```python
from build123d import *

# Parameters (mm, degrees)
BOSS_EXTRUDE1_DEPTH                             = 6.35
SKETCH2_R                                       = 9.525
MOTOR_SHAFT_HOLES_DEPTH                         = 135.10382172
SKETCH3_R                                       = 14.2875
FIRST_BEARING_HOLE_DEPTH                        = 135.10382172
SKETCH4_R                                       = 12.7
PINION_CLEARANCE_DEPTH                          = 3.175
SKETCH5_R                                       = 14.2875
CUT_EXTRUDE1_DEPTH                              = 135.10382172
CBORE_FOR_10_SOCKET_HEAD_CAP_SCREW1_D           = 5.1054
CBORE_FOR_10_SOCKET_HEAD_CAP_SCREW1_CBORE_D     = 9.525
CBORE_FOR_10_SOCKET_HEAD_CAP_SCREW1_CBORE_DEPTH = 4.826
F_10_CLEARANCE_HOLE1_D                          = 5.1054
FILLET1_R                                       = 6.35
SKETCH11_R                                      = 4.7625
CUT_EXTRUDE2_DEPTH                              = 50.8


with BuildPart() as part:
    # Sketch1 → Boss-Extrude1 (new body)
    with BuildSketch(Plane(origin=(0, 0, 0), x_dir=(1, 0, 0), z_dir=(0, 1, 0))):
        Polygon((69.85, -19.05), (69.85, 57.15), (6.35, 114.3), (-6.35, 114.3), (-69.85, 57.15), (-69.85, -19.05), align=None)
    extrude(amount=BOSS_EXTRUDE1_DEPTH)

    # Sketch2 → Motor Shaft Holes (cut, through all)
    with BuildSketch(Plane(origin=(0, 6.35, 0), x_dir=(1, 0, 0), z_dir=(0, 1, 0))):
        with Locations(Location((-34.29, 25.4, 0), (0, 0, 270))):
            Circle(SKETCH2_R)
        with Locations(Location((34.29, 25.4, 0), (0, 0, 270))):
            Circle(SKETCH2_R)
    extrude(amount=-MOTOR_SHAFT_HOLES_DEPTH, mode=Mode.SUBTRACT)

    # Sketch3 → First Bearing Hole (cut, through all)
    with BuildSketch(Plane(origin=(0, 6.35, 0), x_dir=(1, 0, 0), z_dir=(0, 1, 0))):
        with Locations(Location((0, 25.4, 0), (0, 0, 270))):
            Circle(SKETCH3_R)
    extrude(amount=-FIRST_BEARING_HOLE_DEPTH, mode=Mode.SUBTRACT)

    # Sketch4 → Pinion Clearance (cut)
    with BuildSketch(Plane(origin=(0, 6.35, 0), x_dir=(1, 0, 0), z_dir=(0, 1, 0))):
        with Locations(Location((-34.29, 25.4, 0), (0, 0, 270))):
            Circle(SKETCH4_R)
        with Locations(Location((34.29, 25.4, 0), (0, 0, 270))):
            Circle(SKETCH4_R)
    extrude(amount=-PINION_CLEARANCE_DEPTH, mode=Mode.SUBTRACT)

    # Sketch5 → Cut-Extrude1 (cut, through all)
    with BuildSketch(Plane(origin=(0, 6.35, 0), x_dir=(1, 0, 0), z_dir=(0, 1, 0))):
        with Locations(Location((0, 63.5, 0), (0, 0, 270))):
            Circle(SKETCH5_R)
    extrude(amount=-CUT_EXTRUDE1_DEPTH, mode=Mode.SUBTRACT)

    # CBORE for #10 Socket Head Cap Screw1 (through all)
    with Locations(Plane(origin=(0, 6.35, 0), x_dir=(1, 0, 0), z_dir=(0, 1, 0))):
        with Locations((-42.97731164, 49.268192568), (-25.60268836, 1.531807432)):
            cbore_for_10_socket_head_cap_screw1 = CounterBoreHole(CBORE_FOR_10_SOCKET_HEAD_CAP_SCREW1_D / 2, CBORE_FOR_10_SOCKET_HEAD_CAP_SCREW1_CBORE_D / 2, CBORE_FOR_10_SOCKET_HEAD_CAP_SCREW1_CBORE_DEPTH)

    # Mirror1: CBORE for #10 Socket Head Cap Screw1 across plane
    add(cbore_for_10_socket_head_cap_screw1.mirror(Plane(origin=(0, 0, 0), x_dir=(0, 0, 1), z_dir=(1, 0, 0))), mode=Mode.SUBTRACT)

    # #10 Clearance Hole1 (through all)
    with Locations(Plane(origin=(0, 34.925, 19.05), x_dir=(1, 0, 0), z_dir=(0, 1, 0))):
        with Locations((-63.5, 6.35), (63.5, 6.35), (0, 107.95)):
            Hole(F_10_CLEARANCE_HOLE1_D / 2)

    # Fillet1
    fillet1_edges = [part.edges().sort_by_distance(p)[0] for p in [
        (69.85, 3.175, -57.15),
        (69.85, 3.175, 19.05),
        (-69.85, 3.175, 19.05),
        (-69.85, 3.175, -57.15),
        (-6.35, 3.175, -114.3),
        (6.35, 3.175, -114.3),
    ]]
    fillet(fillet1_edges, radius=FILLET1_R)

    # Sketch11 → Cut-Extrude2 (cut)
    with BuildSketch(Plane(origin=(0, 0, 19.05), x_dir=(-1, 0, 0), z_dir=(0, -1, 0))):
        with Locations(Location((-44.45, 85.725, 0), (0, 0, 90))):
            Circle(SKETCH11_R)
        with Locations(Location((44.45, 85.725, 0), (0, 0, 90))):
            Circle(SKETCH11_R)
        with Locations(Location((0, 6.35, 0), (0, 0, 90))):
            Circle(SKETCH11_R)
    extrude(amount=-CUT_EXTRUDE2_DEPTH, mode=Mode.SUBTRACT)


solid = part.part
```
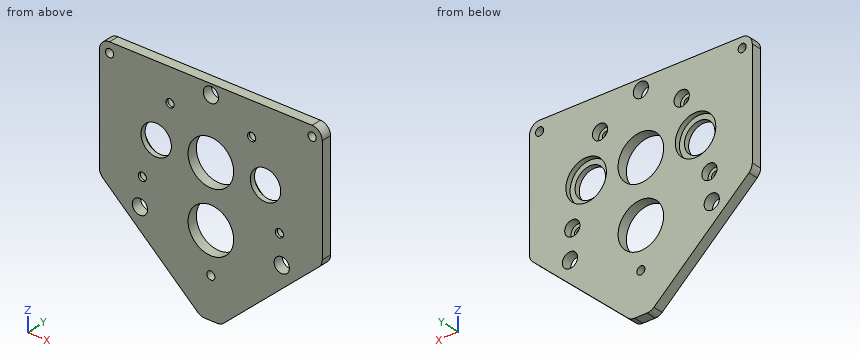
Geometry check sheet. Reference: the model listing, model coordinates, mm. Round coordinates to 2 decimals unless told otherwise and drop trailing zeros. Loops run counter-clockwise (first coordinate to the right, second up) from the corner with the lowest first, then second, coordinate; pieces in that order, holes last. Notation, with made-up numbers: M 62,60.5 L 103,60.5 A28 ccw 103,97.5 Z; hole C -18.75,46 d6. An arc over 180 degrees is marked long. Return JSON: item names as keys, results as strings. Group by question number.
(1) Go/stop test with flat-tipped pins: pin 1 (1 mm diameter, centred on x = 35, y = 1, fed in from -Z) (3 decimals); pin 2 (4.5 mm diameter, centred on x = -25.6, z = -1.53, fed in from -Y); pin 3 (8 mm diameter, centred on x = 25.6, z = -1.53, fed in from +Y); pin 4 (1.5 mm diameter, centred on y = 5, z = -92, fed in from -X). Record where each tip stops, or that it passes through.
(2) Scan lines: line 1 along X through (y, z) = (0.5, 13); line 2 along X through (y, z) = (5, 0); line 3 along X through (y, z) = (4, -26.5). Record each from-to range of solid material in increasing order. Write a range as [from, to].
(3) Section check D-D, the plane x = -34.29. Enter the section's corners in (y, z) (3 decimals), and give its area (3 significant figures).
(4) Section check B-B, the plane x = 0. Enter the section's corners in (y, z), and give its area (3 significant figures).
(5) Section check A-A, the plane z = -25.4. Give the number of separate pieces and of enclosed holes in the cut face, and give its area (3 significant figures).
Data:
{
 "1": {"pin 1": "z = -88.965", "pin 2": "through", "pin 3": "y = 1.52", "pin 4": "x = -31.96"},
 "2": {"line 1": "[-69.84, -66.04], [-60.96, -4.75], [4.75, 60.96], [66.04, 69.84]", "line 2": "[-69.85, -30.11], [-21.09, 21.09], [30.11, 69.85]", "line 3": "[-69.85, -46.94], [-21.64, -14.25], [14.25, 21.64], [46.94, 69.85]"},
 "3": {"outline": "M 0,-89.154 L 6.35,-89.154 L 6.35,-38.1 L 3.175,-38.1 L 3.175,-34.925 L 0,-34.925 Z; M 0,-15.875 L 3.175,-15.875 L 3.175,-12.7 L 6.35,-12.7 L 6.35,19.05 L 0,19.05 Z", "area": "546 mm²"},
 "4": {"outline": "M 0,-114.3 L 6.35,-114.3 L 6.35,-91.45 L 0,-91.45 Z; M 0,-86.35 L 6.35,-86.35 L 6.35,-77.79 L 0,-77.79 Z; M 0,-49.21 L 6.35,-49.21 L 6.35,-39.69 L 0,-39.69 Z; M 0,-11.11 L 6.35,-11.11 L 6.35,7.94 L 0,7.94 Z; M 0,17.46 L 6.35,17.46 L 6.35,19.05 L 0,19.05 Z", "area": "391 mm²"},
 "5": {"separate pieces": "4", "enclosed holes": "0", "area": "423 mm²"}
}
